from build123d import *

# Parameters (mm, degrees)
PAD002_DEPTH  = 4
SKETCH006_R   = 1.5
SKETCH006_R_2 = 0.5
PAD003_DEPTH  = 1.5
FILLET_R      = 0.2


with BuildPart() as part:
    # Sketch005 (on Face1 of CopyPocket002) → Pad002 (new body)
    with BuildSketch(Plane(origin=(0, 0, -1.8), x_dir=(1, 0, 0), z_dir=(0, 0, -1))):
        with BuildLine():
            ThreePointArc((-4.018628, -2.625), (4.8, 0), (-4.018628, 2.625))
            Line((-4.018628, 2.625), (-4.018628, -2.625))
        make_face()
    extrude(amount=PAD002_DEPTH)

    # Sketch006 (on Face4 of Pad002) → Pad003 (join)
    with BuildSketch(Plane(origin=(0, 0, -5.8), x_dir=(1, 0, 0), z_dir=(0, 0, -1))):
        Circle(SKETCH006_R)
        with Locations((0, 4)):
            Circle(SKETCH006_R_2)
        with Locations((0, -4)):
            Circle(SKETCH006_R_2)
    extrude(amount=PAD003_DEPTH)

    # Fillet
    fillet_edges = [part.edges().sort_by_distance(p)[0] for p in [
        (-0.5, -4, -7.3),
        (-0.5, 4, -7.3),
        (-1.5, 0, -7.3),
    ]]
    fillet(fillet_edges, radius=FILLET_R)


solid = part.part
The listing builds one solid part. Answer for the finished solid, in the listing's coordinates (mm). A direction names the side the tool comes from. Coordinates: 2 decimals unless noted, no trailing zeros. Loops run counter-clockwise (first coordinate to the right, second up) from the corner with the lowest first, then second, coordinate; pieces in that order, holes last. Notation, with made-up numbers: (72.25, 75) -> (77.25, 75) arc R8 ccw to (77.25, 81) -> close; hole circle Ø4 at (4, 31.25). An arc over 180 degrees is marked (long way). Answer in a Markdown table with one row per item. Add a question column.
1. The part is cut by section C-C, the plane y = 0. Write down the section's boundary in (x, z), then the cut area to 3 significant figures.
2. Flat-ended cylindrical pins translate along their axes: P1, Ø5, axis at x = 3.5, y = 2.5, coming from the -Z side; P2, Ø1, axis at x = -1.5, z = -6, coming from the -Y side. Find the tip coordinate at first contact, or state that the pin passes through.
3. Consider line 1 (Z direction, x = 3, y = -1.25); line 2 (X direction, y = 0, z = -7); line 3 (X direction, y = -4, z = -4.45). Determine where each line is inside the solid, lowest interval first. Write a range as [from, to].
4. The part is cut by section B-B, the plane z = -6.15. Write down the section's boundary in (x, y).
5. For faces 1 (the flat face through (-4.019, 0, -4)), 2 (the flat face through (1.3, -1.1, -5.8)), determine the directions among +Z, -Z, +X, -X, +Y, -Y from which every point of the face is accessible in a straight line to the end or side of a thin tool.
6. The part is cut by section D-D, the plane y = 4. Write down the section's boundary in (x, z).
7. The part is cut by section A-A, the plane x = 0. Write down the section's boundary in (y, z).
8. Determine the mould class of faces 3 (the cylindrical face through (-0.065, 3.504, -6.441)), 4 (the cylindrical face through (4.797, 0.172, -3.772)), 5 (the flat face through (0, 0, -1.8)) for opening direction Y: +Y half, -Y half, draft (parallel to the pull), parting line (faces both ways), or undercut.
Answer below:
| question | item | result |
|---|---|---|
| 1 | outline | (-4.02, -5.8) -> (-1.5, -5.8) -> (-1.5, -7.1) arc R0.2 ccw to (-1.3, -7.3) -> (1.3, -7.3) arc R0.2 ccw to (1.5, -7.1) -> (1.5, -5.8) -> (4.8, -5.8) -> (4.8, -1.8) -> (-4.02, -1.8) -> close |
| 1 | area | 39.8 mm2 |
| 2 | P1 | z = -5.8 |
| 2 | P2 | y = -4.69 |
| 3 | line 1 | [-5.8, -1.8] |
| 3 | line 2 | [-1.5, 1.5] |
| 3 | line 3 | [-2.65, 2.65] |
| 4 | outline | circle Ø3 at (0, 0); circle Ø1 at (0, -4); circle Ø1 at (0, 4) |
| 5 | face 1 | +Z, -Z, -X, +Y, -Y |
| 5 | face 2 | -Z |
| 6 | outline | (-2.65, -5.8) -> (-0.5, -5.8) -> (-0.5, -7.1) arc R0.2 ccw to (-0.3, -7.3) -> (0.3, -7.3) arc R0.2 ccw to (0.5, -7.1) -> (0.5, -5.8) -> (2.65, -5.8) -> (2.65, -1.8) -> (-2.65, -1.8) -> close |
| 7 | outline | (-4.8, -5.8) -> (-4.5, -5.8) -> (-4.5, -7.1) arc R0.2 ccw to (-4.3, -7.3) -> (-3.7, -7.3) arc R0.2 ccw to (-3.5, -7.1) -> (-3.5, -5.8) -> (-1.5, -5.8) -> (-1.5, -7.1) arc R0.2 ccw to (-1.3, -7.3) -> (1.3, -7.3) arc R0.2 ccw to (1.5, -7.1) -> (1.5, -5.8) -> (3.5, -5.8) -> (3.5, -7.1) arc R0.2 ccw to (3.7, -7.3) -> (4.3, -7.3) arc R0.2 ccw to (4.5, -7.1) -> (4.5, -5.8) -> (4.8, -5.8) -> (4.8, -1.8) -> (-4.8, -1.8) -> close |
| 8 | face 3 | undercut |
| 8 | face 4 | parting line |
| 8 | face 5 | draft |
